Geometry check sheet. Reference: the model listing, model coordinates, mm. Face numbers are marked on the shaded views. Round coordinates to 2 decimals unless told otherwise and drop trailing zeros. Write each loop counter-clockwise with the first axis right and the second up, starting at its lowest first coordinate (ties: lowest second). Pieces come first, ordered by that corner, then holes. Notation, with made-up numbers: (61.25, 54.5) - (108.25, 54.5) arc R28 cw to (108.25, 75.5) - close; hole circle Ø2 at (-39, -23). An arc over 180 degrees is marked (long way). Return JSON: item names as keys, results as strings. Group by question number.
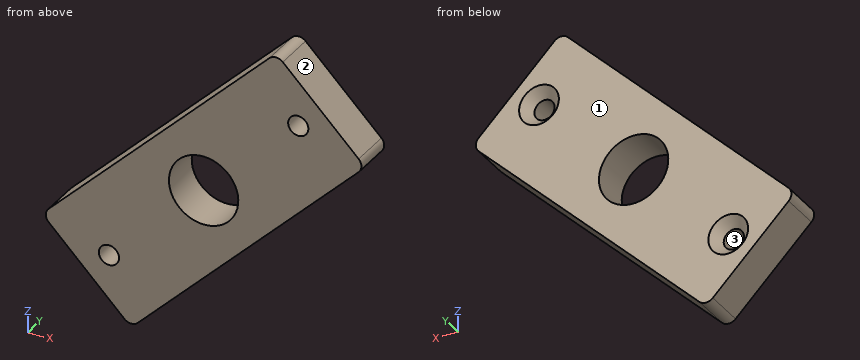
from build123d import *

# Parameters (mm, degrees)
SKETCH2_R                                       = 10.993
BOSS_EXTRUDE1_DEPTH                             = 12.7
CSK_FOR_M6_FLAT_HEAD_MACHINE_SCREW1_D           = 6.4
CSK_FOR_M6_FLAT_HEAD_MACHINE_SCREW1_CSINK_D     = 12.6
CSK_FOR_M6_FLAT_HEAD_MACHINE_SCREW1_CSINK_ANGLE = 90
FILLET1_R                                       = 3


with BuildPart() as part:
    # Sketch2 → Boss-Extrude1 (new body)
    with BuildSketch(Plane(origin=(0, 0, 0), x_dir=(1, 0, 0), z_dir=(0, 1, 0))):
        Polygon((-51.265241636, 22.980970389), (22.980970389, -51.265241636), (51.265241636, -22.980970389), (-22.980970389, 51.265241636), align=None)
        with Locations(Location((0, 0, 0), (0, 0, 270))):
            Circle(SKETCH2_R, mode=Mode.SUBTRACT)
    extrude(amount=-BOSS_EXTRUDE1_DEPTH)

    # CSK for M6 Flat Head Machine Screw1 (through all)
    with Locations(Plane(origin=(-30, 0, -30), x_dir=(0, 0, 1), z_dir=(0, 1, 0))):
        with Locations((0, 0), (60, 60)):
            CounterSinkHole(CSK_FOR_M6_FLAT_HEAD_MACHINE_SCREW1_D / 2, CSK_FOR_M6_FLAT_HEAD_MACHINE_SCREW1_CSINK_D / 2, counter_sink_angle=CSK_FOR_M6_FLAT_HEAD_MACHINE_SCREW1_CSINK_ANGLE)

    # Fillet1
    fillet1_edges = [part.edges().sort_by_distance(p)[0] for p in [
        (-22.980970389, -6.35, -51.265241636),
        (51.265241636, -6.35, 22.980970389),
        (22.980970389, -6.35, 51.265241636),
        (-51.265241636, -6.35, -22.980970389),
    ]]
    fillet(fillet1_edges, radius=FILLET1_R)


solid = part.part
1. Depth check by flat-ended pin: pin 1 Ø3 at (y, z) = (-2.5, 17.5) entering from -X; pin 2 Ø6 at (x, y) = (-37.5, -7) entering from +Z; pin 3 Ø1 at (y, z) = (-6.5, -22) entering from -X. Enter the tip coordinate at first touch or a pass-through.
2. Section check C-C (z = 0). Enter the section's corners in (x, y), and give its area (3 significant figures).
3. Section check A-A (y = -7). Enter the section's corners in (x, z), and give its area (3 significant figures).
4. Section check B-B (x = 0). Enter the section's corners in (y, z), and give its area (3 significant figures).
5. Section check D-D (z = -30). Enter the section's corners in (x, y), and give its area (3 significant figures).
6. Mould release check, pull along X, two halves, no side actions. Record for the marked faces 1, 2 and 3: pulls with the +X half, pulls with the -X half, needs draft (parallel to the pull), parting line crosses it, or undercut.
7. Material ranges on line 1 along Z through (x, y) = (30, -7.5); line 2 along X through (y, z) = (-6.75, 0), recorded low to high.
Result sheet:
{
 "1": {"pin 1": "stops at x = -12.28", "pin 2": "stops at z = -6.22", "pin 3": "stops at x = -49.98"},
 "2": {"outline": "(-28.28, -12.7) - (-10.99, -12.7) - (-10.99, 0) - (-28.28, 0) - close; (10.99, -12.7) - (28.28, -12.7) - (28.28, 0) - (10.99, 0) - close", "area": "439 mm²"},
 "3": {"outline": "(-49.14, -25.1) - (-25.1, -49.14) arc R3 ccw to (-20.86, -49.14) - (49.14, 20.86) arc R3 ccw to (49.14, 25.1) - (25.1, 49.14) arc R3 ccw to (20.86, 49.14) - (-49.14, -20.86) arc R3 ccw to start; hole circle Ø6.4 at (-30, -30); hole circle Ø21.99 at (0, 0); hole circle Ø6.4 at (30, 30)", "area": "3,750 mm²"},
 "4": {"outline": "(-12.7, -28.28) - (0, -28.28) - (0, -10.99) - (-12.7, -10.99) - close; (-12.7, 10.99) - (0, 10.99) - (0, 28.28) - (-12.7, 28.28) - close", "area": "439 mm²"},
 "5": {"outline": "(-44.25, -12.7) - (-33.2, -12.7) - (-33.2, -3.1) - (-36.3, 0) - (-44.25, 0) - close; (-26.8, -12.7) - (-1.72, -12.7) - (-1.72, 0) - (-23.7, 0) - (-26.8, -3.1) - close", "area": "449 mm²"},
 "6": {"face 1": "needs draft", "face 2": "pulls with the +X half", "face 3": "undercut"},
 "7": {"line 1": "z = 1.72 to 26.8, 33.2 to 44.25", "line 2": "x = -28.28 to -10.99, 10.99 to 28.28"}
}
